```python
from build123d import *

# Parameters (mm, degrees)
F1_DEPTH = 2.54
F0_W     = 12.7
F0_H     = 27.94
F0_R     = 0.762
F2_DEPTH = 3.81
F3_DEPTH = 3.81
F4_R     = 0.762


# Not quite as in the source:
# - a feature names something its author has since deleted; it is built from what else it names


with BuildPart() as f1:
    # F0 (on Front) → F1 (new body)
    with BuildSketch(Plane.XZ):
        Polygon((0, 54.1968159378), (-57.15, 26.67), (57.15, 26.67), align=None)
        Polygon((-57.15, -13.97), (-8.382, -13.97), (-8.382, 16.002), (8.382, 16.002), (8.382, -13.97), (57.15, -13.97), (57.15, 26.67), (-57.15, 26.67), align=None)
    extrude(amount=F1_DEPTH)



with BuildPart() as f1b:
    # F0 (on Front) → F1, piece 2 (new body)
    with BuildSketch(Plane.XZ):
        Rectangle(F0_W, F0_H)
        with Locations((-4.064, 1.27)):
            Circle(F0_R, mode=Mode.SUBTRACT)
    extrude(amount=F1_DEPTH)


with BuildPart() as f1_1:
    add(f1.part)

    add(f1b.part)  # F2 merges F1b
    # F0 (on Front) → F2 (join)
    with BuildSketch(Plane.XZ):
        Polygon((-6.35, -13.97), (-6.35, 13.97), (6.35, 13.97), (6.35, -13.97), (8.382, -13.97), (8.382, 16.002), (-8.382, 16.002), (-8.382, -13.97), align=None)
    extrude(amount=F2_DEPTH)

    # F0 (on Front) → F3 (join)
    with BuildSketch(Plane.XZ):
        with Locations((-4.064, 1.27)):
            Circle(F0_R)
    extrude(amount=F3_DEPTH)

    # F4
    f4_edges = [f1_1.edges().sort_by_distance(p)[0] for p in [
        (-4.826, -3.81, 1.27),
    ]]
    fillet(f4_edges, radius=F4_R)


solid = f1_1.part
```
Read the model definition and answer for the solid it produces. Units are mm, in the model's axes. Give positions to 0.01 mm unless a question says otherwise; leave off trailing zeros. Loops run counter-clockwise (first coordinate to the right, second up) from the corner with the lowest first, then second, coordinate; pieces in that order, holes last.
Item 1: The part is cut by section A-A (z = -4.5). Write down the section's boundary in (x, y).
Item 2: The mould has two halves that part along X. Classify faces 1 (the flat face through (-28.17, -1.25, 40.63)), 2 (the flat face through (-1, -1, -13.97)), 3 (the flat face through (0, -2.54, 0)): released by +X, released by -X, zero draft, split by the parting line, or undercut.
Item 3: Each of these flat-tipped pins is pushed along its axis until it touches: pin 1 Ø1 at (y, z) = (-3, 7) entering from -X; pin 2 Ø2 at (x, y) = (23, -3) entering from +Z; pin 3 Ø6 at (x, z) = (-41.5, 40) entering from -Y; pin 4 Ø1.4 at (x, y) = (-4, -3.5) entering from +Z. Where does it stop, or does it pass through?
Item 4: The part is cut by section B-B (y = -1.2). Write down the section's boundary in (x, z), and give its area (3 significant figures).
Item 5: Find the intervals of material crossed by line 1 along X through (y, z) = (-3.55, -3.5); line 2 along Y through (x, z) = (-41.5, 24.5); line 3 along Z through (x, y) = (-47, -0.85), in increasing order.
Item 6: The part is cut by section C-C (x = 34.5). Write down the section's boundary in (y, z), and give its area (3 significant figures).
Item 7: The part is cut by section D-D (z = 21). Write down the section's boundary in (x, y).
Taken from the geometry:
1. outline: (-57.15, -2.54) - (-8.38, -2.54) - (-8.38, -3.81) - (-6.35, -3.81) - (-6.35, -2.54) - (6.35, -2.54) - (6.35, -3.81) - (8.38, -3.81) - (8.38, -2.54) - (57.15, -2.54) - (57.15, 0) - (-57.15, 0) - close
2. face 1: released by -X
2. face 2: zero draft
2. face 3: undercut
3. pin 1: stops at x = -57.15
3. pin 2: stops at z = 43.55
3. pin 3: passes through
3. pin 4: stops at z = 16
4. outline: (-57.15, -13.97) - (57.15, -13.97) - (57.15, 26.67) - (0, 54.2) - (-57.15, 26.67) - close
4. area: 6,220 mm2
5. line 1: x = -8.38 to -6.35, 6.35 to 8.38
5. line 2: y = -2.54 to 0
5. line 3: z = -13.97 to 31.56
6. outline: (-2.54, -13.97) - (0, -13.97) - (0, 37.58) - (-2.54, 37.58) - close
6. area: 131 mm2
7. outline: (-57.15, -2.54) - (57.15, -2.54) - (57.15, 0) - (-57.15, 0) - close
